Verification items for the finished model (mm, model axes). A direction names the side the tool comes from. Round coordinates to 2 decimals unless told otherwise and drop trailing zeros. Loops run counter-clockwise (first coordinate to the right, second up) from the corner with the lowest first, then second, coordinate; pieces in that order, holes last. Notation, with made-up numbers: (60, 28.25) -> (111, 28.25) arc R27 ccw to (111, 45.25) -> close; hole circle Ø8 at (-2, -28). An arc over 180 degrees is marked (long way). Write item = value, one per line.
```python
from build123d import *

# Parameters (mm, degrees)
F1_DEPTH = 6.4


with BuildPart() as f1:
    # F0 (on Top) → F1 (new body)
    with BuildSketch(Plane.XY):
        with BuildLine():
            Line((1.327045, 0), (23.223624, 0))
            Line((23.223624, 0), (22.276235, 18.077263))
            ThreePointArc((22.276235, 18.077263), (21.655685, 19.423339), (20.278976, 19.972591))
            Line((20.278976, 19.972591), (17.176905, 19.972591))
            Line((17.176905, 19.972591), (12.883583, 5))
            Line((12.883583, 5), (6.923761, 6.708952))
            Line((6.923761, 6.708952), (8.577585, 12.476522))
            Line((8.577585, 12.476522), (6.591801, 12.476522))
            ThreePointArc((6.591801, 12.476522), (4.184541, 11.671064), (2.746754, 9.579071))
            Line((2.746754, 9.579071), (0.365783, 1.275637))
            ThreePointArc((0.365783, 1.275637), (0.528409, 0.398185), (1.327045, 0))
        make_face()
    extrude(amount=F1_DEPTH)


solid = f1.part
```
(1) Sectioned sample at B-B, the plane z = 2. Record the cut outline in (x, y), and give its area (3 significant figures).
Filled sheet:
outline = (0.37, 1.28) arc R1 ccw to (1.33, 0) -> (23.22, 0) -> (22.28, 18.08) arc R2 ccw to (20.28, 19.97) -> (17.18, 19.97) -> (12.88, 5) -> (6.92, 6.71) -> (8.58, 12.48) -> (6.59, 12.48) arc R4 ccw to (2.75, 9.58) -> close
area = 265 mm2
(2) Draft check along X on faces 1 (the face through (22.757, 8.912, 3.155)), 2 (the face through (15.06, 12.59, 3.16)), 3 (the face through (14, 8, 0)), 4 (the face through (9.95, 5.84, 3.16)). Enter one of: released by +X, released by -X, zero draft, split by the parting line, or undercut.
Filled sheet:
face_1 = released by +X
face_2 = undercut
face_3 = zero draft
face_4 = undercut
(3) Set-up check for faces 5 (the face through (12, 0, 3)), 6 (the face through (7.74, 9.55, 3.16)), 7 (the face through (8, 12.477, 3)): record each of +Z, -Z, +X, -X, +Y, -Y from which the full face is reachable in a straight line by a thin tool's end or side.
Filled sheet:
face_5 = +Z, -Z, +X, -X, -Y
face_6 = +Z, -Z
face_7 = +Z, -Z, -X, +Y
(4) Go/stop test with flat-tipped pins: pin 1 Ø3 at (x, y) = (12, 7.5) entering from -Z; pin 2 Ø2 at (x, z) = (7.5, 4.5) entering from +Y; pin 3 Ø2 at (y, z) = (13, 5.5) entering from +X; pin 4 Ø1 at (y, z) = (6.5, 2) entering from +X. Record where each tip stops, or that it passes through.
Filled sheet:
pin_1 = through
pin_2 = 12.48
pin_3 = 22.59
pin_4 = 22.91
(5) Material ranges on probe 1 along X at (y, z) = (9, 6.25); probe 2 along X at (y, z) = (12, 4.5); probe 3 along Y at (x, z) = (11.25, 0.75), recorded low to high. Write a range as from..to.
Filled sheet:
probe_1 = 2.58..7.58, 14.03..22.75
probe_2 = 4.7..8.44, 14.89..22.59
probe_3 = 0..5.47
(6) Sectioned sample at A-A, the plane y = 12. Record the cut outline in (x, z).
Filled sheet:
outline = (4.7, 0) -> (8.44, 0) -> (8.44, 6.4) -> (4.7, 6.4) -> close; (14.89, 0) -> (22.59, 0) -> (22.59, 6.4) -> (14.89, 6.4) -> close
(7) Sectioned sample at D-D, the plane x = 10.75. Record the cut outline in (y, z).
Filled sheet:
outline = (0, 0) -> (5.61, 0) -> (5.61, 6.4) -> (0, 6.4) -> close
(8) Sectioned sample at C-C, the plane y = 7.25. Record the cut outline in (x, z), and give its area (3 significant figures).
Filled sheet:
outline = (2.08, 0) -> (7.08, 0) -> (7.08, 6.4) -> (2.08, 6.4) -> close; (13.53, 0) -> (22.84, 0) -> (22.84, 6.4) -> (13.53, 6.4) -> close
area = 91.6 mm2
